Check sheet for the modelled part. Datum: model origin and axes. Units: mm. A direction names the side the tool comes from. Coordinates: 2 decimals unless noted, no trailing zeros. Write each loop counter-clockwise with the first axis right and the second up, starting at its lowest first coordinate (ties: lowest second). Pieces come first, ordered by that corner, then holes. Notation, with made-up numbers: (-12, 21.25) -> (44, 21.25) arc R21 cw to (44, 56.25) -> close; hole circle Ø4 at (53.5, 50.5). An arc over 180 degrees is marked (long way). One line per item, written item: value. Start each with the question number.
1) Gauge pin test, flat ends, axial feed: P1, Ø8, axis at y = 4.5, z = -200, coming from the -X side; P2, Ø24, axis at x = -327, z = -109.5, coming from the +Y side. Record the tip position at first contact, or that the pin passes through.
2) Sectioned sample at A-A on x = -169.5. Enter the section's corners in (y, z), plus the area to 3 significant figures.
3) Draft check along Y on faces 1 (the flat face through (-101, 10, -137)), 2 (the flat face through (-150, -35, -115)), 3 (the flat face through (-101, 5, 0)). Enter one of: +Y half, -Y half, draft (parallel to the pull), parting line (faces both ways), or undercut.
4) Sectioned sample at C-C on x = -93.5. Enter the section's corners in (y, z), plus the area to 3 significant figures.
5) Scan lines: line 1 along Y through (x, z) = (-163.5, -237); line 2 along Z through (x, y) = (-281, -74); line 3 along X through (y, z) = (0.5, -242). Record each from-to range of solid material in increasing order. Write a range as [from, to].
6) Sectioned sample at B-B on y = -84.5. Enter the section's corners in (x, z), plus the area to 3 significant figures.
7) Set-up check for faces 4 (the flat face through (-120, -49, -115)), 5 (the flat face through (-257, -73, -100)), 6 (the flat face through (-297, -100, -115)), 7 (the flat face through (-101, 5, -270.285)), 8 (the flat face through (-257, -73, -130)): record each of +Z, -Z, +X, -X, +Y, -Y from which the full face is reachable in a straight line by a thin tool's end or side.
```python
from build123d import *

# Parameters (mm, degrees)
SKETCH1_W      = 200
SKETCH1_H      = 270.285174582
EXTRUDE1_DEPTH = 10
SKETCH2_W      = 30
SKETCH2_H      = 30
EXTRUDE2_DEPTH = 100
SKETCH3_W      = 30
SKETCH3_H      = 30
EXTRUDE3_DEPTH = 330


with BuildPart() as part:
    # Sketch1 → Extrude1 (new body)
    with BuildSketch(Plane(origin=(0, 0, 0), x_dir=(1, 0, 0), z_dir=(0, 1, 0))):
        with Locations((-100, 135.142587291)):
            Rectangle(SKETCH1_W, SKETCH1_H)
    extrude(amount=EXTRUDE1_DEPTH)

    # Sketch2 → Extrude2 (add)
    with BuildSketch(Plane.XZ):
        with Locations((-135, -115)):
            Rectangle(SKETCH2_W, SKETCH2_H)
    extrude(amount=EXTRUDE2_DEPTH)

    # Sketch3 → Extrude3 (add)
    with BuildSketch(Plane.ZY.offset(150)):
        with Locations((-115, -85)):
            Rectangle(SKETCH3_W, SKETCH3_H)
    extrude(amount=EXTRUDE3_DEPTH)


solid = part.part
```
Answers:
1. P1: stops at x = -200
1. P2: stops at y = -70
2. outline: (-100, -130) -> (-70, -130) -> (-70, -100) -> (-100, -100) -> close; (0, -270.29) -> (10, -270.29) -> (10, 0) -> (0, 0) -> close
2. area: 3,600 mm2
3. face 1: +Y half
3. face 2: undercut
3. face 3: draft
4. outline: (0, -270.29) -> (10, -270.29) -> (10, 0) -> (0, 0) -> close
4. area: 2,700 mm2
5. line 1: y = [0, 10]
5. line 2: z = [-130, -100]
5. line 3: x = [-200, 0]
6. outline: (-480, -130) -> (-120, -130) -> (-120, -100) -> (-480, -100) -> close
6. area: 10,800 mm2
7. face 4: +Z, -Z, +X, -Y
7. face 5: +Z, +X, -X, -Y
7. face 6: +Z, -Z, +X, -X, -Y
7. face 7: -Z, +X, -X, +Y, -Y
7. face 8: -Z, +X, -X, -Y
